from build123d import *

# Parameters (mm, degrees)
SKETCH1_W           = 13.7
SKETCH1_H           = 42
BOSS_EXTRUDE1_DEPTH = 6.35
SKETCH2_W           = 13.7
SKETCH2_H           = 18
BOSS_EXTRUDE2_DEPTH = 26.65
CUT_EXTRUDE1_DEPTH  = 14.7
SKETCH4_R           = 2.75
CUT_EXTRUDE2_DEPTH  = 7.35


with BuildPart() as part:
    # Sketch1 → Boss-Extrude1 (new body)
    with BuildSketch(Plane(origin=(0, 0, 0), x_dir=(1, 0, 0), z_dir=(0, 1, 0))):
        Rectangle(SKETCH1_W, SKETCH1_H)
    extrude(amount=BOSS_EXTRUDE1_DEPTH)

    # Sketch2 → Boss-Extrude2 (add)
    with BuildSketch(Plane(origin=(0, 6.35, 0), x_dir=(1, 0, 0), z_dir=(0, 1, 0))):
        Rectangle(SKETCH2_W, SKETCH2_H)
    extrude(amount=BOSS_EXTRUDE2_DEPTH)

    # Sketch3 → Cut-Extrude1 (cut, through all)
    with BuildSketch(Plane.ZY.offset(6.85)):
        with BuildLine():
            Line((-0.6, 24), (-0.6, 33))
            Line((-0.6, 33), (0.6, 33))
            Line((0.6, 33), (0.6, 24))
            ThreePointArc((0.6, 24), (0, 16.045256013), (-0.6, 24))
        make_face()
    extrude(amount=-CUT_EXTRUDE1_DEPTH, mode=Mode.SUBTRACT)

    # Sketch4 → Cut-Extrude2 (cut, through all)
    with BuildSketch(Plane(origin=(0, 6.35, 0), x_dir=(1, 0, 0), z_dir=(0, 1, 0))):
        with Locations((0, -15.75)):
            Circle(SKETCH4_R)
    cut_extrude2 = extrude(amount=-CUT_EXTRUDE2_DEPTH, mode=Mode.SUBTRACT)

    # Mirror1: Cut-Extrude2 across plane
    add(cut_extrude2.mirror(Plane.XY), mode=Mode.SUBTRACT)


solid = part.part
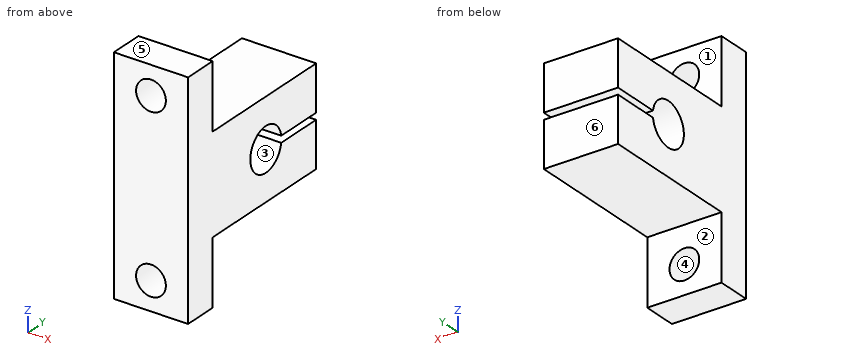
The listing builds one solid part. Answer for the finished solid, in the listing's coordinates (mm). Face numbers are marked on the shaded views. A direction names the side the tool comes from. Round coordinates to 2 decimals unless told otherwise and drop trailing zeros. Order: outer loops, then holes, each group sorted by start corner. A loop starts at its lowest first (then second) coordinate and runs counter-clockwise, first axis right, second up. Notation, with made-up numbers: (-38.5, 36.5) -> (-21.5, 36.5) arc R19 cw to (-21.5, 68.5) -> close; hole circle Ø4 at (-34.5, 85). An arc over 180 degrees is marked (long way). Write each question's results on one line, items separated by ' | '. Start each with the question number.
Q1. Find section A-A (x = 0). Determine the outline of the cut face in (y, z), then the cut area to 3 significant figures.
Q2. Find section B-B (z = 15.75). Determine the outline of the cut face in (x, y), then the cut area to 3 significant figures.
Q3. Which of the six approach directions +Z, -Z, +X, -X, +Y, -Y give full straight-line access (tool end or side, diameter ignored) to the marked faces 1, 2 and 3?
Q4. Find section D-D (y = 4). Determine the outline of the cut face in (x, z), then the cut area to 3 significant figures.
Q5. Each of these flat-tipped pins is pushed along its axis until it touches: pin 1 (7 mm diameter, centred on x = 2.5, y = 28, fed in from -Z); pin 2 (1 mm diameter, centred on x = -0.5, z = 13.5, fed in from +Y); pin 3 (7 mm diameter, centred on x = 0, y = 20.5, fed in from +Z). Where does it stop, or does it pass through?
Q6. The mould has two halves that part along Z. Classify the marked faces 4, 5 and 6: pulls with the +Z half, pulls with the -Z half, needs draft (parallel to the pull), parting line crosses it, or undercut.
Q7. Straight lines are drawn through the part: probe 1 along Z at (x, y) = (0, 2.5); probe 2 along Z at (x, y) = (5, 27); probe 3 along X at (y, z) = (2.75, -15.75). For each, find the intervals that lie inside material, in ascending order. Write a range as from..to.
Q8. Find section C-C (y = 25). Determine the outline of the cut face in (x, z).
Worked answers:
1) outline: (0, -21) -> (6.35, -21) -> (6.35, -18.5) -> (0, -18.5) -> close; (0, -13) -> (6.35, -13) -> (6.35, -9) -> (33, -9) -> (33, -0.6) -> (24, -0.6) arc R4 cw (long way) to (24, 0.6) -> (33, 0.6) -> (33, 9) -> (6.35, 9) -> (6.35, 13) -> (0, 13) -> close; (0, 18.5) -> (6.35, 18.5) -> (6.35, 21) -> (0, 21) -> close | area: 616 mm2
2) outline: (-6.85, 0) -> (-2.75, 0) -> (-2.75, 6.35) -> (-6.85, 6.35) -> close; (2.75, 0) -> (6.85, 0) -> (6.85, 6.35) -> (2.75, 6.35) -> close | area: 52.1 mm2
3) face 1: +Z, +X, -X, +Y | face 2: -Z, +X, -X, +Y | face 3: +X, -X
4) outline: (-6.85, -21) -> (6.85, -21) -> (6.85, 21) -> (-6.85, 21) -> close; hole circle Ø5.5 at (0, -15.75); hole circle Ø5.5 at (0, 15.75) | area: 528 mm2
5) pin 1: stops at z = -9 | pin 2: stops at y = 6.35 | pin 3: stops at z = 9
6) face 4: undercut | face 5: pulls with the +Z half | face 6: needs draft
7) probe 1: z = -21..-18.5, -13..13, 18.5..21 | probe 2: z = -9..-0.6, 0.6..9 | probe 3: x = -6.85..-2.75, 2.75..6.85
8) outline: (-6.85, -9) -> (6.85, -9) -> (6.85, -0.6) -> (-6.85, -0.6) -> close; (-6.85, 0.6) -> (6.85, 0.6) -> (6.85, 9) -> (-6.85, 9) -> close
